Work out the finished part from the listing and answer in its coordinate system (mm). A direction names the side the tool comes from. Coordinates: 2 decimals unless noted, no trailing zeros. Order: outer loops, then holes, each group sorted by start corner. A loop starts at its lowest first (then second) coordinate and runs counter-clockwise, first axis right, second up. Notation, with made-up numbers: (29.5, 14.5) -> (82.5, 14.5) arc R11 ccw to (82.5, 20.5) -> close; hole circle Ø9 at (-37, 12.25). An arc over 180 degrees is marked (long way). Write item = value, one per line. Start each with the question number.
Q1. Which of the six approach directions +Z, -Z, +X, -X, +Y, -Y give full straight-line access (tool end or side, diameter ignored) to faces 1 (the flat face through (70.35, 3.13, -98.85)), 2 (the flat face through (-117, 3, 7)), 3 (the flat face through (-64.53, 3.131, -97.844)), 4 (the cylindrical face through (-107.874, 3.131, -63.153)), 5 (the cylindrical face through (107.874, 3.131, 63.153))?
Q2. For a pull along Z with two mould halves and no side action, classify faces 6 (the flat face through (-58.257, 3.131, -106.004)), 7 (the flat face through (70.3, 3.13, 98.76)), 8 (the flat face through (-117, 3, -7)), 9 (the flat face through (29.9, 3, 55)) as +Z half, -Z half, draft (parallel to the pull), parting line (faces both ways), or undercut.
Q3. The part is cut by section C-C, the plane z = 6.5. Determine the outline of the cut face in (x, y).
Q4. Flat-ended cylindrical pins translate along their axes: pin 1 (1.9 mm diameter, centred on y = 2, z = -7, fed in from -X); pin 2 (3 mm diameter, centred on y = 4, z = 51, fed in from +X); pin 3 (3 mm diameter, centred on x = -81, y = 5, fed in from -Z). Find the tip coordinate at first contact, or state that the pin passes through.
Q5. The part is cut by section D-D, the plane x = -91.5. Determine the outline of the cut face in (y, z).
Q6. Straight lines are drawn through the part: L1, parallel to Z at x = 27.7, y = 3 (3 decimals); L2, parallel to Z at x = -27.7, y = 3.25 (3 decimals); L3, parallel to Z at x = 50.5, y = 2.5. For each, find the intervals that lie inside material, in ascending order. Write a range as from..to.
Q7. The part is cut by section B-B, the plane y = 5.25. Count the separate pieces of the cut face and the enclosed holes in it, plus the area to 3 significant figures.
Q8. The part is cut by section A-A, the plane x = 12. Determine the outline of the cut face in (y, z).
```python
from build123d import *

# Parameters (mm, degrees)
SKETCH1_R           = 2
SKETCH1_W           = 39.8
SKETCH1_H           = 19.8
BOSS_EXTRUDE1_DEPTH = 6.35
SKETCH3_R           = 3.175
CUT_EXTRUDE1_DEPTH  = 6.35


with BuildPart() as part:
    # Sketch1 → Boss-Extrude1 (new body)
    with BuildSketch(Plane(origin=(0, 0, 0), x_dir=(1, 0, 0), z_dir=(0, 1, 0))):
        with BuildLine():
            Line((-124.469875874, 11.5), (-117, 11.5))
            Line((-117, 11.5), (-117, 2.55))
            Line((-117, 2.55), (-124.973987293, 2.55))
            ThreePointArc((-124.973987293, 2.55), (-125, 0), (-124.973987293, -2.55))
            Line((-124.973987293, -2.55), (-117, -2.55))
            Line((-117, -2.55), (-117, -11.5))
            Line((-117, -11.5), (-124.469875874, -11.5))
            ThreePointArc((-124.469875874, -11.5), (-108.253175473, -62.5), (-72.19423008, -102.044074512))
            Line((-72.19423008, -102.044074512), (-68.459292144, -95.574972243))
            Line((-68.459292144, -95.574972243), (-60.70836478, -100.049972243))
            Line((-60.70836478, -100.049972243), (-64.695358426, -106.955647808))
            ThreePointArc((-64.695358426, -106.955647808), (-62.5, -108.253175473), (-60.278628867, -109.505647808))
            Line((-60.278628867, -109.505647808), (-56.29163522, -102.599972243))
            Line((-56.29163522, -102.599972243), (-48.540707856, -107.074972243))
            Line((-48.540707856, -107.074972243), (-52.275645793, -113.544074512))
            ThreePointArc((-52.275645793, -113.544074512), (0, -125), (52.275645793, -113.544074512))
            Line((52.275645793, -113.544074512), (48.540707856, -107.074972243))
            Line((48.540707856, -107.074972243), (56.29163522, -102.599972243))
            Line((56.29163522, -102.599972243), (60.278628867, -109.505647808))
            ThreePointArc((60.278628867, -109.505647808), (62.5, -108.253175473), (64.695358426, -106.955647808))
            Line((64.695358426, -106.955647808), (60.70836478, -100.049972243))
            Line((60.70836478, -100.049972243), (68.459292144, -95.574972243))
            Line((68.459292144, -95.574972243), (72.19423008, -102.044074512))
            ThreePointArc((72.19423008, -102.044074512), (108.253175473, -62.5), (124.469875874, -11.5))
            Line((124.469875874, -11.5), (117, -11.5))
            Line((117, -11.5), (117, -2.55))
            Line((117, -2.55), (124.973987293, -2.55))
            ThreePointArc((124.973987293, -2.55), (125, 0), (124.973987293, 2.55))
            Line((124.973987293, 2.55), (117, 2.55))
            Line((117, 2.55), (117, 11.5))
            Line((117, 11.5), (124.469875874, 11.5))
            ThreePointArc((124.469875874, 11.5), (108.253175473, 62.5), (72.19423008, 102.044074512))
            Line((72.19423008, 102.044074512), (68.459292144, 95.574972243))
            Line((68.459292144, 95.574972243), (60.70836478, 100.049972243))
            Line((60.70836478, 100.049972243), (64.695358426, 106.955647808))
            ThreePointArc((64.695358426, 106.955647808), (62.5, 108.253175473), (60.278628867, 109.505647808))
            Line((60.278628867, 109.505647808), (56.29163522, 102.599972243))
            Line((56.29163522, 102.599972243), (48.540707856, 107.074972243))
            Line((48.540707856, 107.074972243), (52.275645793, 113.544074512))
            ThreePointArc((52.275645793, 113.544074512), (0, 125), (-52.275645793, 113.544074512))
            Line((-52.275645793, 113.544074512), (-48.540707856, 107.074972243))
            Line((-48.540707856, 107.074972243), (-56.29163522, 102.599972243))
            Line((-56.29163522, 102.599972243), (-60.278628867, 109.505647808))
            ThreePointArc((-60.278628867, 109.505647808), (-62.5, 108.253175473), (-64.695358426, 106.955647808))
            Line((-64.695358426, 106.955647808), (-60.70836478, 100.049972243))
            Line((-60.70836478, 100.049972243), (-68.459292144, 95.574972243))
            Line((-68.459292144, 95.574972243), (-72.19423008, 102.044074512))
            ThreePointArc((-72.19423008, 102.044074512), (-108.253175473, 62.5), (-124.469875874, 11.5))
        make_face()
        with Locations((34.4, 60)):
            Circle(SKETCH1_R, mode=Mode.SUBTRACT)
        with Locations((34.4, 50)):
            Circle(SKETCH1_R, mode=Mode.SUBTRACT)
        with Locations((-14.4, 60)):
            Circle(SKETCH1_R, mode=Mode.SUBTRACT)
        with Locations((-14.4, 50)):
            Circle(SKETCH1_R, mode=Mode.SUBTRACT)
        with Locations((-14.4, -60)):
            Circle(SKETCH1_R, mode=Mode.SUBTRACT)
        with Locations((-14.4, -50)):
            Circle(SKETCH1_R, mode=Mode.SUBTRACT)
        with Locations((34.4, -60)):
            Circle(SKETCH1_R, mode=Mode.SUBTRACT)
        with Locations((34.4, -50)):
            Circle(SKETCH1_R, mode=Mode.SUBTRACT)
        with Locations((10, 55)):
            Rectangle(SKETCH1_W, SKETCH1_H, mode=Mode.SUBTRACT)
        with Locations((10, -55)):
            Rectangle(SKETCH1_W, SKETCH1_H, mode=Mode.SUBTRACT)
    extrude(amount=BOSS_EXTRUDE1_DEPTH)

    # Sketch3 → Cut-Extrude1 (cut)
    with BuildSketch(Plane(origin=(0, 6.35, 0), x_dir=(1, 0, 0), z_dir=(0, 1, 0))):
        with Locations((-27.7, -102.7)):
            Circle(SKETCH3_R)
        with Locations((27.7, -102.7)):
            Circle(SKETCH3_R)
        with Locations((27.7, 102.7)):
            Circle(SKETCH3_R)
        with Locations((-27.7, 102.7)):
            Circle(SKETCH3_R)
    extrude(amount=-CUT_EXTRUDE1_DEPTH, mode=Mode.SUBTRACT)


solid = part.part
```
Model answer:
q1.face_1 = -Z, +Y, -Y
q1.face_2 = -X, +Y, -Y
q1.face_3 = +Y, -Y
q1.face_4 = -Z, -X, +Y, -Y
q1.face_5 = +Z, +X, +Y, -Y
q2.face_6 = -Z half
q2.face_7 = +Z half
q2.face_8 = undercut
q2.face_9 = undercut
q3.outline = (-117, 0) -> (117, 0) -> (117, 6.35) -> (-117, 6.35) -> close
q4.pin_1 = -117
q4.pin_2 = 114.78
q4.pin_3 = -96.46
q5.outline = (0, -85.16) -> (6.35, -85.16) -> (6.35, 85.16) -> (0, 85.16) -> close
q6.L1 = -121.892..-105.875, -99.525..-64.9, -45.1..45.1, 64.9..99.525, 105.875..121.892
q6.L2 = -121.892..-105.875, -99.525..99.525, 105.875..121.892
q6.L3 = -114.34..-110.47, -105.94..105.94, 110.47..114.34
q7.separate_pieces = 1
q7.enclosed_holes = 14
q7.area = 46,400 mm2
q8.outline = (0, -124.42) -> (6.35, -124.42) -> (6.35, -64.9) -> (0, -64.9) -> close; (0, -45.1) -> (6.35, -45.1) -> (6.35, 45.1) -> (0, 45.1) -> close; (0, 64.9) -> (6.35, 64.9) -> (6.35, 124.42) -> (0, 124.42) -> close
